Read the model definition and answer for the solid it produces. Units are mm, in the model's axes. Face numbers are marked on the shaded views. A direction names the side the tool comes from. Give positions to 0.01 mm unless a question says otherwise; leave off trailing zeros. Write each loop counter-clockwise with the first axis right and the second up, starting at its lowest first coordinate (ties: lowest second). Pieces come first, ordered by that corner, then holes. Notation, with made-up numbers: (86, -20) - (119, -20) arc R17 cw to (119, 2) - close; hole circle Ø3 at (6.25, 14.25). An arc over 180 degrees is marked (long way). Answer as CSV lines item,"result".
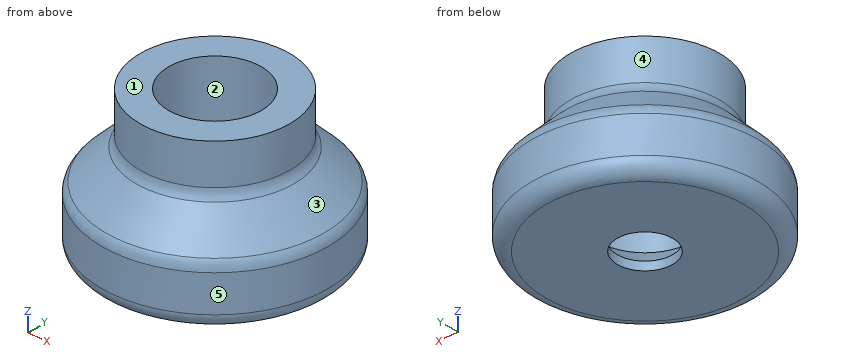
```python
from build123d import *


with BuildPart() as f1:
    # F0 (on Front) → F1 (revolve)
    with BuildSketch(Plane.XZ):
        with BuildLine():
            Line((1.956549, 0.6), (1.956549, 0))
            Line((1.956549, 0), (7, 0))
            ThreePointArc((7, 0), (7.707107, 0.292893), (8, 1))
            Line((8, 1), (8, 3.585786))
            ThreePointArc((8, 3.585786), (7.92388, 3.96847), (7.707107, 4.292893))
            Line((7.707107, 4.292893), (5.567893, 6.432107))
            ThreePointArc((5.567893, 6.432107), (5.35112, 6.75653), (5.275, 7.139214))
            Line((5.275, 7.139214), (5.275, 10))
            Line((5.275, 10), (3.275, 10))
            Line((3.275, 10), (3.275, 1.918451))
            Line((3.275, 1.918451), (1.956549, 0.6))
        make_face()
    revolve(axis=Axis((0, 0, 7.164844), (0, 0, 1)))


solid = f1.part
```
(1) A cutting plane is placed at D-D (z = 7.5). Write down the section's boundary in (x, y) (3 decimals), and give its area (3 significant figures).
Worked out:
outline,"circle Ø10.55 at (0, 0); hole circle Ø6.55 at (0, 0)"
area,"53.7 mm^2"
(2) A cutting plane is placed at C-C (z = 4.5). Write down the section's boundary in (x, y) (3 decimals).
Worked out:
outline,"circle Ø15 at (0, 0); hole circle Ø6.55 at (0, 0)"
(3) The mould has two halves that part along X. Classify the marked faces 1, 2 and 3: +X half, -X half, draft (parallel to the pull), parting line (faces both ways), or undercut.
Worked out:
face 1,"draft"
face 2,"undercut"
face 3,"parting line"
(4) For the marked faces 4 and 5, determine the directions among +Z, -Z, +X, -X, +Y, -Y from which every point of the face is accessible in a straight line to the end or side of a thin tool.
Worked out:
face 4,"+Z"
face 5,"+Z, -Z"
(5) Find the intervals of material crossed by L1, parallel to Y at x = 0, z = 5 (3 decimals); L2, parallel to Y at x = 0, z = 0.25; L3, parallel to X at y = 1.75, z = 1.5, in increasing order.
Worked out:
L1,"y = -7 to -3.275, 3.275 to 7"
L2,"y = -7.66 to -1.96, 1.96 to 7.66"
L3,"x = -7.81 to -2.26, 2.26 to 7.81"
(6) A cutting plane is placed at A-A (y = 0). Write down the section's boundary in (x, z) (3 decimals), and give its area (3 significant figures).
Worked out:
outline,"(-8, 1) arc R1 ccw to (-7, 0) - (-1.957, 0) - (-1.957, 0.6) - (-3.275, 1.918) - (-3.275, 10) - (-5.275, 10) - (-5.275, 7.139) arc R1 cw to (-5.568, 6.432) - (-7.707, 4.293) arc R1 ccw to (-8, 3.586) - close; (1.957, 0) - (7, 0) arc R1 ccw to (8, 1) - (8, 3.586) arc R1 ccw to (7.707, 4.293) - (5.568, 6.432) arc R1 cw to (5.275, 7.139) - (5.275, 10) - (3.275, 10) - (3.275, 1.918) - (1.957, 0.6) - close"
area,"72.1 mm^2"
(7) Each of these flat-tipped pins is pushed along its axis until it touches: P1, Ø1, axis at x = 1, z = 2.5, coming from the -Y side; P2, Ø6, axis at y = -4.5, z = 9, coming from the -X side; P3, Ø8, axis at x = -3, y = -3, coming from the -Z side; P4, Ø6, axis at y = 3, z = 5.5, coming from the +X side. Where does it stop, or does it pass through?
Worked out:
P1,"stops at y = -7.98"
P2,"stops at x = -5.06"
P3,"stops at z = 0"
P4,"stops at x = 7.97"
